Source: CAD feature listing. Evaluate the final solid. Frame: model axes, mm. Coordinates: 2 decimals unless noted, no trailing zeros. Write each loop counter-clockwise with the first axis right and the second up, starting at its lowest first coordinate (ties: lowest second). Pieces come first, ordered by that corner, then holes. Notation, with made-up numbers: (-12, 82) -> (2, 82) arc R13 ccw to (2, 96) -> close; hole circle Ø6 at (53, 74). An arc over 180 degrees is marked (long way). Write item = value, one per line.
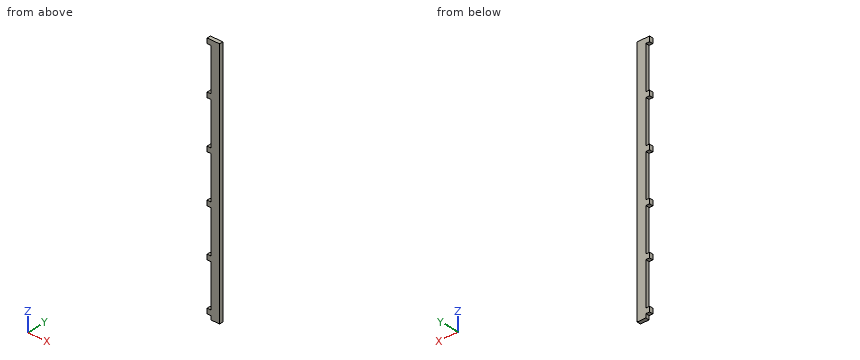
Autodesk Inventor part; units mm, degrees
ref_plane "YZ Plane" through (0, 0, 0) normal (1, 0, 0) x (0, 1, 0)
ref_plane "XZ Plane" through (0, 0, 0) normal (0, 1, 0) x (-1, 0, 0)
ref_plane "XY Plane" through (0, 0, 0) normal (0, 0, 1) x (1, 0, 0)
sketch "Sketch1" plane through (0, 0, 0) normal (0, 1, 0) x (-1, 0, 0)
  line L0 (-5, 3.5) -> (-5, -3.5)
  line L1 (-5, -3.5) -> (2, -3.5)
  line L2 (5, -0.5) -> (5, 3.5)
  line L3 (5, 3.5) -> (2, 3.5)
  line L4 (5, -0.5) -> (2, -0.5)
  line L5 (2, -0.5) -> (2, -3.5)
  line L6 (5, 37.5) -> (2, 37.5)
  line L7 (5, 37.5) -> (5, 41.5)
  line L8 (5, 41.5) -> (2, 41.5)
  line L9 (5, 75.5) -> (2, 75.5)
  line L10 (5, 75.5) -> (5, 79.5)
  line L11 (5, 79.5) -> (2, 79.5)
  line L12 (5, 113.5) -> (2, 113.5)
  line L13 (5, 113.5) -> (5, 117.5)
  line L14 (5, 117.5) -> (2, 117.5)
  line L15 (5, 151.5) -> (2, 151.5)
  line L16 (5, 151.5) -> (5, 155.5)
  line L17 (5, 155.5) -> (2, 155.5)
  line L18 (5, 189.5) -> (2, 189.5)
  line L19 (5, 189.5) -> (5, 193.5)
  line L20 (5, 193.5) -> (2, 193.5)
  line L21 (2, 3.5) -> (2, 37.5)
  line L22 (2, 41.5) -> (2, 75.5)
  line L23 (2, 79.5) -> (2, 113.5)
  line L24 (2, 117.5) -> (2, 151.5)
  line L25 (2, 155.5) -> (2, 189.5)
  line L26 (-5, 193.5) -> (-5, 3.5)
  line L27 (2, 193.5) -> (-5, 193.5)
  point P0 (0, 0)
  dimension "d10" = 3
  dimension "d18" = 38
extrude "Extrusion1" add sketch "Sketch1" along normal blind 3
properties part number "steun" material "Wood (Maple)"
1) Cut plane B-B, the plane z = 83.5. Output: boundary loops of the cut face in (x, y), and give its area (3 significant figures).
Answer block:
outline = (-2, 0) -> (5, 0) -> (5, 3) -> (-2, 3) -> close
area = 21.0 mm2
2) First-contact query: pin 1 Ø0.9 at (y, z) = (1, 18.5) entering from -X; pin 2 Ø0.9 at (x, y) = (-4, 1) entering from -Z. Flat tips, straight axial feed; report the tip coordinate or a pass-through.
Answer block:
pin_1 = -2
pin_2 = -0.5
3) Cut plane A-A, the plane y = 1.75. Output: boundary loops of the cut face in (x, z).
Answer block:
outline = (-5, -0.5) -> (-2, -0.5) -> (-2, -3.5) -> (5, -3.5) -> (5, 193.5) -> (-5, 193.5) -> (-5, 189.5) -> (-2, 189.5) -> (-2, 155.5) -> (-5, 155.5) -> (-5, 151.5) -> (-2, 151.5) -> (-2, 117.5) -> (-5, 117.5) -> (-5, 113.5) -> (-2, 113.5) -> (-2, 79.5) -> (-5, 79.5) -> (-5, 75.5) -> (-2, 75.5) -> (-2, 41.5) -> (-5, 41.5) -> (-5, 37.5) -> (-2, 37.5) -> (-2, 3.5) -> (-5, 3.5) -> close
4) Material intervals for probe 1 along Z at (x, y) = (-3.25, 2.1); probe 2 along X at (y, z) = (1.8, 74), sorted ascending. Write a range as [from, to].
Answer block:
probe_1 = [-0.5, 3.5], [37.5, 41.5], [75.5, 79.5], [113.5, 117.5], [151.5, 155.5], [189.5, 193.5]
probe_2 = [-2, 5]
